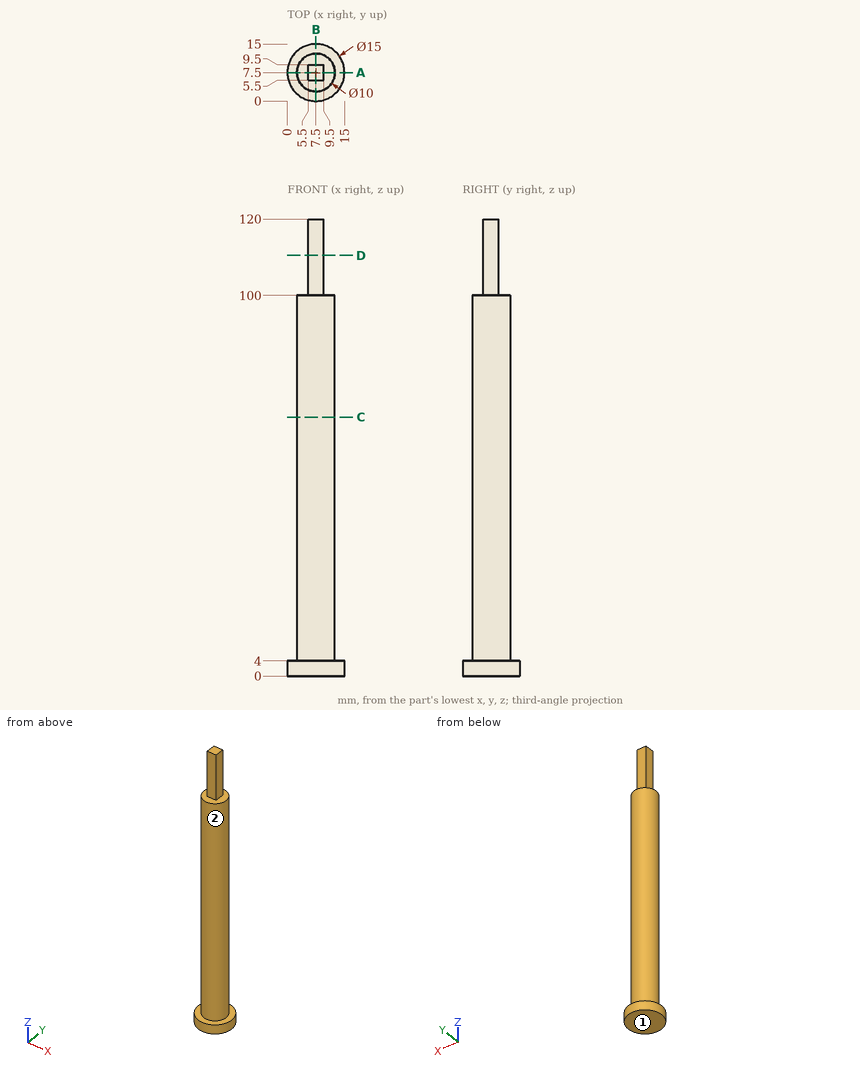
Geometry: see drawing. Coordinates: mm, zero at the bounding-box minimum. A direction names the side the tool comes from. Give positions to 0.01 mm unless a question says otherwise; leave off trailing zeros. Loops run counter-clockwise (first coordinate to the right, second up) from the corner with the lowest first, then second, coordinate; pieces in that order, holes last. Notation, with made-up numbers: M -11,65.5 L 35,65.5 A28 cw 35,100.5 Z; hole C 27.25,51 d1. An arc over 180 degrees is marked long. Answer as CSV lines item,"result". Start each with the question number.
1. Section D-D on z = 110.5. Return loops of the section in (x, y), plus the area to 3 significant figures.
2. Section C-C on z = 68. Return loops of the section in (x, y), plus the area to 3 significant figures.
3. Section A-A on y = 7.5. Return loops of the section in (x, z), plus the area to 3 significant figures.
4. Line query: L1, parallel to Z at x = 11.75, y = 4.5; L2, parallel to Z at x = 7.5, y = 11; L3, parallel to X at y = 6.5, z = 110.5. Output: solid intervals per line, ascending.
5. Pin query (flat end, axial travel): P1, Ø4.5, axis at x = 6.5, z = 107, coming from the -Y side; P2, Ø1.5, axis at y = 10, z = 49, coming from the -X side; P3, Ø3, axis at y = 10.5, z = 90, coming from the -X side. Return the tip coordinate at first contact, or that it passes through.
6. Reachability of the marked faces 1 and 2 from +Z, -Z, +X, -X, +Y, -Y: full face, straight path, thin tool, end or side. Return the list, or none.
Computed values:
1,outline,"M 5.5,5.5 L 9.5,5.5 L 9.5,9.5 L 5.5,9.5 Z"
1,area,"16.0 mm²"
2,outline,"C 7.5,7.5 d10"
2,area,"78.5 mm²"
3,outline,"M 0,0 L 15,0 L 15,4 L 12.5,4 L 12.5,100 L 9.5,100 L 9.5,120 L 5.5,120 L 5.5,100 L 2.5,100 L 2.5,4 L 0,4 Z"
3,area,"1,100 mm²"
4,L1,"z = 0 to 4"
4,L2,"z = 0 to 100"
4,L3,"x = 5.5 to 9.5"
5,P1,"stops at y = 5.5"
5,P2,"stops at x = 2.82"
5,P3,"stops at x = 2.73"
6,face 1,"-Z, +X, -X, +Y, -Y"
6,face 2,"+Z"
